```python
from build123d import *

# Parameters (mm, degrees)
SKETCH1_R           = 3
BOSS_EXTRUDE1_DEPTH = 15
CUT_EXTRUDE2_START  = -12
CUT_EXTRUDE2_DEPTH  = 12
SKETCH3_R           = 10
BOSS_EXTRUDE2_DEPTH = 4
CUT_EXTRUDE3_REACH  = 25.685
SKETCH5_R           = 16
BOSS_EXTRUDE3_DEPTH = 27
SKETCH6_R           = 15
BOSS_EXTRUDE4_DEPTH = 60
SKETCH9_R           = 1.5
CUT_EXTRUDE4_DEPTH  = 5


with BuildPart() as part:
    # Sketch1 → Boss-Extrude1 (new body)
    with BuildSketch(Plane.XY):
        Circle(SKETCH1_R)
    extrude(amount=BOSS_EXTRUDE1_DEPTH)

    # Sketch2 → Cut-Extrude2 (cut)
    with BuildSketch(Plane.XY.offset(15).offset(CUT_EXTRUDE2_START)):
        with BuildLine():
            Line((1.658312395, -2.5), (-1.658312395, -2.5))
            ThreePointArc((-1.658312395, -2.5), (0, -3), (1.658312395, -2.5))
        make_face()
    extrude(amount=CUT_EXTRUDE2_DEPTH, mode=Mode.SUBTRACT)

    # Sketch3 → Boss-Extrude2 (add)
    with BuildSketch(Plane(origin=(0, 0, 0), x_dir=(-1, 0, 0), z_dir=(0, 0, -1))):
        Circle(SKETCH3_R)
    extrude(amount=BOSS_EXTRUDE2_DEPTH)

    # Sketch4 → Cut-Extrude3 (cut, up to next)
    with BuildSketch(Plane(origin=(0, 0, -4), x_dir=(-1, 0, 0), z_dir=(0, 0, -1)), mode=Mode.PRIVATE) as cut_extrude3_sk1:
        with BuildLine():
            Line((-3.281754029, -9.446168032), (-9.446168032, -3.281754029))
            ThreePointArc((-9.446168032, -3.281754029), (-7.071067812, -7.071067812), (-3.281754029, -9.446168032))
        make_face()
    cut_extrude3_tool1 = extrude(cut_extrude3_sk1.sketch, amount=-CUT_EXTRUDE3_REACH, mode=Mode.PRIVATE) & part.part
    # Sketch4 → Cut-Extrude3 (cut, up to next)
    with BuildSketch(Plane(origin=(0, 0, -4), x_dir=(-1, 0, 0), z_dir=(0, 0, -1)), mode=Mode.PRIVATE) as cut_extrude3_sk2:
        with BuildLine():
            ThreePointArc((9.446168032, 3.281754029), (7.071067812, 7.071067812), (3.281754029, 9.446168032))
            Line((3.281754029, 9.446168032), (9.446168032, 3.281754029))
        make_face()
    cut_extrude3_tool2 = extrude(cut_extrude3_sk2.sketch, amount=-CUT_EXTRUDE3_REACH, mode=Mode.PRIVATE) & part.part
    add(cut_extrude3_tool1.solids().sort_by_distance((6.648052, -6.648052, -4))[0], mode=Mode.SUBTRACT)
    add(cut_extrude3_tool2.solids().sort_by_distance((-6.648052, 6.648052, -4))[0], mode=Mode.SUBTRACT)

    # Sketch5 → Boss-Extrude3 (add)
    with BuildSketch(Plane(origin=(0, 0, -4), x_dir=(-1, 0, 0), z_dir=(0, 0, -1))):
        Circle(SKETCH5_R)
    extrude(amount=BOSS_EXTRUDE3_DEPTH)

    # Sketch6 → Boss-Extrude4 (add)
    with BuildSketch(Plane(origin=(0, 0, -31), x_dir=(-1, 0, 0), z_dir=(0, 0, -1))):
        Circle(SKETCH6_R)
    extrude(amount=BOSS_EXTRUDE4_DEPTH)

    # Sketch9 → Cut-Extrude4 (cut)
    with BuildSketch(Plane.XY.offset(-4)):
        with Locations((0, 13)):
            Circle(SKETCH9_R)
        with Locations((13, 0)):
            Circle(SKETCH9_R)
        with Locations((0, -13)):
            Circle(SKETCH9_R)
        with Locations((-13, 0)):
            Circle(SKETCH9_R)
    extrude(amount=-CUT_EXTRUDE4_DEPTH, mode=Mode.SUBTRACT)


solid = part.part
```
Model file for the job. Use its own axes, mm. A direction names the side the tool comes from. Round coordinates to 2 decimals unless told otherwise and drop trailing zeros. Write each loop counter-clockwise with the first axis right and the second up, starting at its lowest first coordinate (ties: lowest second). Pieces come first, ordered by that corner, then holes. Notation, with made-up numbers: (88.25, -1.75) -> (119.25, -1.75) arc R26 ccw to (119.25, 15.25) -> close; hole circle Ø4 at (-16.75, -17.75). An arc over 180 degrees is marked (long way). Answer as CSV lines item,"result".
1. Slice it at B-B, the plane y = 0. List the corners of the cut face in (x, z), plus the area to 3 significant figures.
Resolved:
outline,"(-16, -31) -> (-15, -31) -> (-15, -91) -> (15, -91) -> (15, -31) -> (16, -31) -> (16, -4) -> (14.5, -4) -> (14.5, -9) -> (11.5, -9) -> (11.5, -4) -> (10, -4) -> (10, 0) -> (3, 0) -> (3, 15) -> (-3, 15) -> (-3, 0) -> (-10, 0) -> (-10, -4) -> (-11.5, -4) -> (-11.5, -9) -> (-14.5, -9) -> (-14.5, -4) -> (-16, -4) -> close"
area,"2,800 mm²"
2. Pin check, flat tips, straight feed: pin 1 Ø3.5 at (x, y) = (-0.5, 13.5) entering from +Z; pin 2 Ø12 at (y, z) = (7, -44) entering from +X; pin 3 Ø1.5 at (x, y) = (-12.5, -0.5) entering from +Z. Stop position of each tip, or through.
Resolved:
pin 1,"z = -4"
pin 2,"x = 14.97"
pin 3,"z = -9"
3. Slice it at D-D, the plane x = -5. List the corners of the cut face in (y, z), plus the area to 3 significant figures.
Resolved:
outline,"(-15.2, -31) -> (-14.14, -31) -> (-14.14, -91) -> (14.14, -91) -> (14.14, -31) -> (15.2, -31) -> (15.2, -4) -> (7.73, -4) -> (7.73, 0) -> (-8.66, 0) -> (-8.66, -4) -> (-15.2, -4) -> close"
area,"2,580 mm²"
4. Slice it at C-C, the plane z = -1. List the corners of the cut face in (x, y).
Resolved:
outline,"(-9.45, 3.28) arc R10 ccw to (3.28, -9.45) -> (9.45, -3.28) arc R10 ccw to (-3.28, 9.45) -> close"
5. Slice it at A-A, the plane x = 0. List the corners of the cut face in (y, z), plus the area to 3 significant figures.
Resolved:
outline,"(-16, -31) -> (-15, -31) -> (-15, -91) -> (15, -91) -> (15, -31) -> (16, -31) -> (16, -4) -> (14.5, -4) -> (14.5, -9) -> (11.5, -9) -> (11.5, -4) -> (10, -4) -> (10, 0) -> (3, 0) -> (3, 15) -> (-2.5, 15) -> (-2.5, 3) -> (-3, 3) -> (-3, 0) -> (-10, 0) -> (-10, -4) -> (-11.5, -4) -> (-11.5, -9) -> (-14.5, -9) -> (-14.5, -4) -> (-16, -4) -> close"
area,"2,800 mm²"
6. Tool access for faces 1 (the face through (6.32, -6.41, -2.03)), 2 (the face through (14.985, 0.66, -60.58)), 3 (the face through (7, -7, -4)): list every direction of +Z, -Z, +X, -X, +Y, -Y with a clear straight run to the whole face (end or side of a thin tool).
Resolved:
face 1,"+Z, +X, -Y"
face 2,"-Z"
face 3,"+Z"
7. Drill centre lines: line 1 (Y direction, x = 0, z = -6.7); line 2 (Z direction, x = 2.5, y = 9); line 3 (Z direction, x = -9.5, y = -7). Where is each one in solid material? Low to high.
Resolved:
line 1,"-16 to -14.5, -11.5 to 11.5, 14.5 to 16"
line 2,"-91 to 0"
line 3,"-91 to -4"
8. Mould opens along X. For faces 4 (the face through (-6.32, 6.41, -2.03)), 5 (the face through (0, -2.5, 9)), 6 (the face through (11.5, 0.07, -6.46)) say: +X half, -X half, draft (parallel to the pull), parting line (faces both ways), or undercut.
Resolved:
face 4,"-X half"
face 5,"draft"
face 6,"undercut"
